from build123d import *

# Parameters (mm, degrees)
SKETCH1_W           = 83
SKETCH1_H           = 59
BOSS_EXTRUDE1_DEPTH = 2
FILLET1_R           = 3
SKETCH2_R           = 1.5
CUT_EXTRUDE1_DEPTH  = 2
SKETCH4_W           = 66
SKETCH4_H           = 44
BOSS_EXTRUDE2_DEPTH = 18


with BuildPart() as part:
    # Sketch1 → Boss-Extrude1 (new body)
    with BuildSketch(Plane.XY):
        with Locations((41.5, 29.5)):
            Rectangle(SKETCH1_W, SKETCH1_H)
    extrude(amount=BOSS_EXTRUDE1_DEPTH)

    # Fillet1
    fillet1_edges = [part.edges().sort_by_distance(p)[0] for p in [
        (0, 59, 1),
        (83, 59, 1),
        (83, 0, 1),
        (0, 0, 1),
    ]]
    fillet(fillet1_edges, radius=FILLET1_R)

    # Sketch2 → Cut-Extrude1 (cut)
    with BuildSketch(Plane.XY.offset(2)):
        with Locations((3.5, 55.5)):
            Circle(SKETCH2_R)
        with Locations((79.5, 55.5)):
            Circle(SKETCH2_R)
    cut_extrude1 = extrude(amount=-CUT_EXTRUDE1_DEPTH, mode=Mode.SUBTRACT)

    # Mirror1: Cut-Extrude1 across plane
    add(cut_extrude1.mirror(Plane(origin=(0, 29.5, 0), x_dir=(0, 0, 1), z_dir=(0, -1, 0))), mode=Mode.SUBTRACT)

    # Sketch4 → Boss-Extrude2 (add)
    with BuildSketch(Plane.XY.offset(2)):
        with Locations((41.5, 29.5)):
            Rectangle(SKETCH4_W, SKETCH4_H)
    extrude(amount=BOSS_EXTRUDE2_DEPTH)


solid = part.part
Read the model definition and answer for the solid it produces. Units are mm, in the model's axes. A direction names the side the tool comes from. Give positions to 0.01 mm unless a question says otherwise; leave off trailing zeros. Loops run counter-clockwise (first coordinate to the right, second up) from the corner with the lowest first, then second, coordinate; pieces in that order, holes last. Notation, with made-up numbers: (54.25, 83.25) - (96.25, 83.25) arc R18 cw to (96.25, 107.25) - close; hole circle Ø6 at (-2, 80). An arc over 180 degrees is marked (long way). Answer as CSV lines item,"result". Start each with the question number.
1) Find section C-C (z = 11.25). Write down the section's boundary in (x, y).
2) Find section B-B (x = 15.5). Write down the section's boundary in (y, z).
3) Straight lines are drawn through the part: L1, parallel to Y at x = 3.5, z = 0.95; L2, parallel to X at y = 3.5, z = 0.7; L3, parallel to Z at x = 8, y = 25. For each, find the intervals that lie inside material, in ascending order. Write a range as from..to.
4) Each of these flat-tipped pins is pushed along its axis until it touches: pin 1 Ø1.5 at (y, z) = (29, 16) entering from -X; pin 2 Ø5 at (x, y) = (3.5, 55.5) entering from +Z; pin 3 Ø4 at (x, z) = (15, 8) entering from +Y. Where does it stop, or does it pass through?
5) Which of the six approach directions +Z, -Z, +X, -X, +Y, -Y give full straight-line access (tool end or side, diameter ignored) to faces 5 (the face through (74.5, 29, 11)), 6 (the face through (41, 7.5, 11)), 7 (the face through (41, 51.5, 11)), 8 (the face through (8.5, 29, 11))?
6) Find section A-A (y = 29). Write down the section's boundary in (x, z).
7) Determine the mould class of faces 1 (the face through (41, 59, 1)), 2 (the face through (0, 29, 1)), 3 (the face through (4.886, 54.925, 1.014)), 4 (the face through (82.1, 0.86, 1.01)) for opening direction X: released by +X, released by -X, zero draft, split by the parting line, or undercut.
Findings below:
1,outline,"(8.5, 7.5) - (74.5, 7.5) - (74.5, 51.5) - (8.5, 51.5) - close"
2,outline,"(0, 0) - (59, 0) - (59, 2) - (51.5, 2) - (51.5, 20) - (7.5, 20) - (7.5, 2) - (0, 2) - close"
3,L1,"0..2, 5..54, 57..59"
3,L2,"0..2, 5..78, 81..83"
3,L3,"0..2"
4,pin 1,"x = 8.5"
4,pin 2,"z = 2"
4,pin 3,"y = 51.5"
5,face 5,"+Z, +X, +Y, -Y"
5,face 6,"+Z, +X, -X, -Y"
5,face 7,"+Z, +X, -X, +Y"
5,face 8,"+Z, -X, +Y, -Y"
6,outline,"(0, 0) - (83, 0) - (83, 2) - (74.5, 2) - (74.5, 20) - (8.5, 20) - (8.5, 2) - (0, 2) - close"
7,face 1,"zero draft"
7,face 2,"released by -X"
7,face 3,"undercut"
7,face 4,"released by +X"
